Input: dimensioned drawing with shaded views. Units: mm. Origin: part minimum x, y, z. A direction names the side the tool comes from. Round coordinates to 2 decimals unless told otherwise and drop trailing zeros. Loops run counter-clockwise (first coordinate to the right, second up) from the corner with the lowest first, then second, coordinate; pieces in that order, holes last. Notation, with made-up numbers: M -12.5,-34.75 L 36.5,-34.75 A13 cw 36.5,-19.75 Z; hole C -35.75,-31 d1. An arc over 180 degrees is marked long. Return JSON: item names as keys, results as strings.
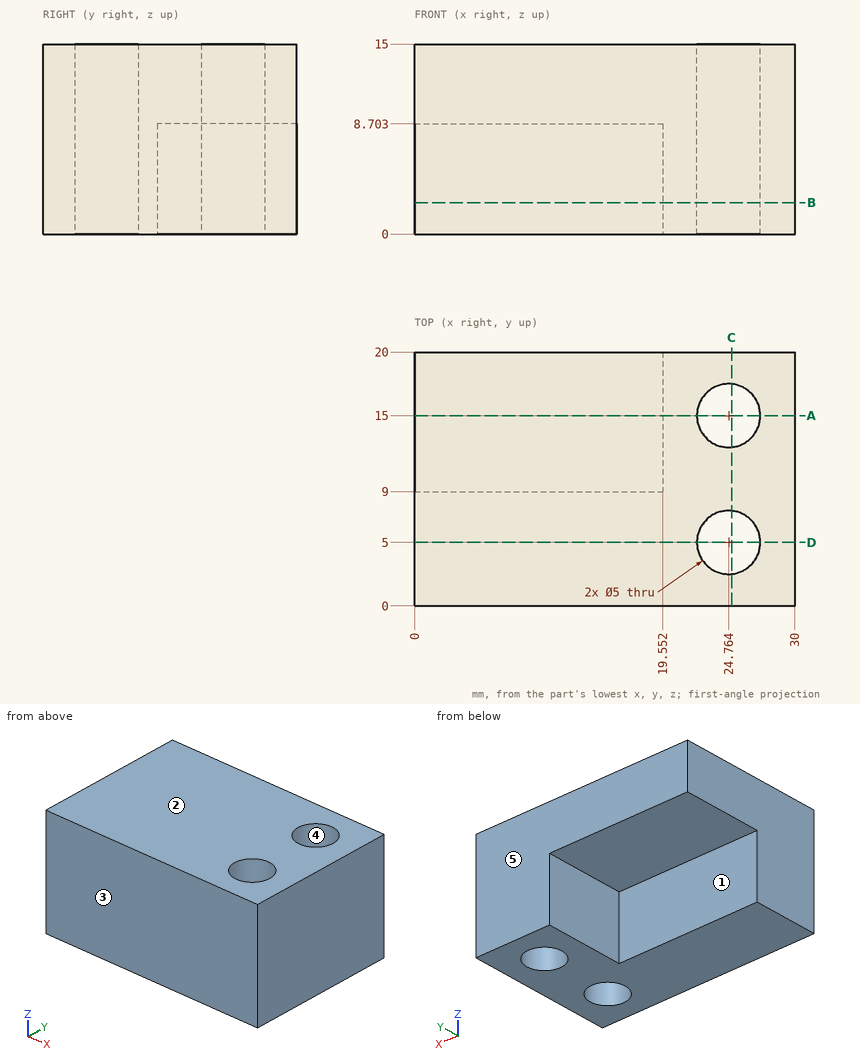
Q1. Pull-direction query (Y, two-part tool) for the marked faces 3, 4 and 5; classes: pulls with the +Y half, pulls with the -Y half, needs draft (parallel to the pull), parting line crosses it, or undercut.
Determined:
{"face 3": "pulls with the -Y half", "face 4": "undercut", "face 5": "pulls with the +Y half"}
Q2. Section query B-B (z = 2.5). Output: boundary loops of the cut face in (x, y).
Determined:
{"outline": "M 0,0 L 30,0 L 30,20 L 19.55,20 L 19.55,9 L 0,9 Z; hole C 24.76,5 d5; hole C 24.76,15 d5"}
Q3. Section query D-D (y = 5). Output: boundary loops of the cut face in (x, z).
Determined:
{"outline": "M 0,0 L 22.26,0 L 22.26,15 L 0,15 Z; M 27.26,0 L 30,0 L 30,15 L 27.26,15 Z"}
Q4. Pin query (flat end, axial travel): pin 1 (4.5 mm diameter, centred on x = 7.5, z = 3, fed in from +Y); pin 2 (3.5 mm diameter, centred on x = 9, y = 12.5, fed in from -Z); pin 3 (3 mm diameter, centred on x = 24.76, y = 15, fed in from -Z); pin 4 (4.5 mm diameter, centred on y = 17, z = 5.5, fed in from -X). Return the tip coordinate at first contact, or that it passes through.
Determined:
{"pin 1": "stops at y = 9", "pin 2": "stops at z = 8.7", "pin 3": "passes through", "pin 4": "stops at x = 19.55"}
Q5. Material intervals for L1, parallel to X at y = 5, z = 9.75; L2, parallel to Y at x = 24, z = 5.5; L3, parallel to Y at x = 25, z = 3, sorted ascending.
Determined:
{"L1": "x = 0 to 22.26, 27.26 to 30", "L2": "y = 0 to 2.62, 7.38 to 12.62, 17.38 to 20", "L3": "y = 0 to 2.51, 7.49 to 12.51, 17.49 to 20"}
Q6. Section query A-A (y = 15). Output: boundary loops of the cut face in (x, z), plus the area to 3 significant figures.
Determined:
{"outline": "M 0,8.7 L 19.55,8.7 L 19.55,0 L 22.26,0 L 22.26,15 L 0,15 Z; M 27.26,0 L 30,0 L 30,15 L 27.26,15 Z", "area": "205 mm^2"}
Q7. Section query C-C (x = 25). Output: boundary loops of the cut face in (y, z), plus the area to 3 significant figures.
Determined:
{"outline": "M 0,0 L 2.51,0 L 2.51,15 L 0,15 Z; M 7.49,0 L 12.51,0 L 12.51,15 L 7.49,15 Z; M 17.49,0 L 20,0 L 20,15 L 17.49,15 Z", "area": "151 mm^2"}
Q8. Reachability of the marked faces 1 and 2 from +Z, -Z, +X, -X, +Y, -Y: full face, straight path, thin tool, end or side. Return the list, or none.
Determined:
{"face 1": "-Z, -X, +Y", "face 2": "+Z, +X, -X, +Y, -Y"}
